from build123d import *

# Parameters (mm, degrees)
F0_R     = 1.524
F1_DEPTH = 3.175


with BuildPart() as f1:
    # F0 (on Top) → F1 (new body)
    with BuildSketch(Plane.XY):
        with BuildLine():
            Line((-6.35, 25.4), (6.35, 25.4))
            Line((6.35, 25.4), (6.35, 44.45))
            ThreePointArc((6.35, 44.45), (4.490128, 48.940128), (0, 50.8))
            ThreePointArc((0, 50.8), (-4.490128, 48.940128), (-6.35, 44.45))
            Line((-6.35, 44.45), (-6.35, 25.4))
        make_face()
        with BuildLine():
            Line((6.35, -19.05), (6.35, 25.4))
            Line((6.35, 25.4), (-6.35, 25.4))
            Line((-6.35, 25.4), (-6.35, -19.05))
            ThreePointArc((-6.35, -19.05), (-4.490128, -23.540128), (0, -25.4))
            ThreePointArc((0, -25.4), (4.490128, -23.540128), (6.35, -19.05))
        make_face()
        with Locations((0, -19.05)):
            Circle(F0_R, mode=Mode.SUBTRACT)
        with Locations((0, 19.05)):
            Circle(F0_R, mode=Mode.SUBTRACT)
    extrude(amount=F1_DEPTH)


solid = f1.part
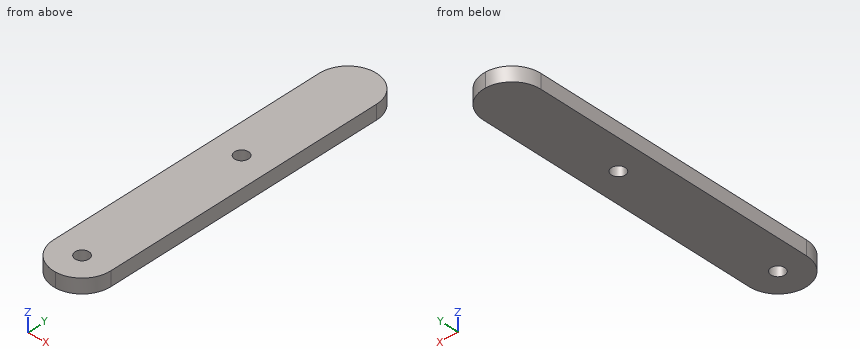
The listing builds one solid part. Answer for the finished solid, in the listing's coordinates (mm). Round coordinates to 2 decimals unless told otherwise and drop trailing zeros. Loops run counter-clockwise (first coordinate to the right, second up) from the corner with the lowest first, then second, coordinate; pieces in that order, holes last. Notation, with made-up numbers: M 24.25,48 L 75.25,48 A14 cw 75.25,66 Z; hole C 33.25,5.25 d7. An arc over 180 degrees is marked long. Return JSON: item names as keys, results as strings.
Q1. Find section D-D, the plane x = -5.5. Determine the outline of the cut face in (y, z) (3 decimals).
Results list:
{"outline": "M -22.224,0 L 47.624,0 L 47.624,3.175 L -22.224,3.175 Z"}
Q2. Find section A-A, the plane y = 19.05. Determine the outline of the cut face in (x, z) (3 decimals), plus the area to 3 significant figures.
Results list:
{"outline": "M -6.35,0 L -1.524,0 L -1.524,3.175 L -6.35,3.175 Z; M 1.524,0 L 6.35,0 L 6.35,3.175 L 1.524,3.175 Z", "area": "30.6 mm2"}
Q3. Find section B-B, the plane z = 1.85. Determine the outline of the cut face in (x, y), plus the area to 3 significant figures.
Results list:
{"outline": "M -6.35,-19.05 A6.35 ccw 6.35,-19.05 L 6.35,44.45 A6.35 ccw -6.35,44.45 Z; hole C 0,-19.05 d3.05; hole C 0,19.05 d3.05", "area": "919 mm2"}
Q4. Find section C-C, the plane x = 5.25. Determine the outline of the cut face in (y, z) (3 decimals).
Results list:
{"outline": "M -22.622,0 L 48.022,0 L 48.022,3.175 L -22.622,3.175 Z"}
Q5. Each of these flat-tipped pins is pushed along its axis until it touches: pin 1 Ø2.5 at (x, y) = (0, -19.05) entering from +Z; pin 2 Ø1.5 at (x, z) = (1.5, 2) entering from -Y. Where does it stop, or does it pass through?
Results list:
{"pin 1": "passes through", "pin 2": "stops at y = -25.36"}
Q6. Find the intervals of material crossed by line 1 along Y through (x, z) = (-5, 2.4); line 2 along Y through (x, z) = (-4.75, 0.7), in increasing order. Write a range as from..to.
Results list:
{"line 1": "y = -22.96..48.36", "line 2": "y = -23.26..48.66"}
